Geometry check sheet. Reference: the model listing, model coordinates, mm. A direction names the side the tool comes from. Round coordinates to 2 decimals unless told otherwise and drop trailing zeros. Loops run counter-clockwise (first coordinate to the right, second up) from the corner with the lowest first, then second, coordinate; pieces in that order, holes last. Notation, with made-up numbers: (57.25, -37) -> (80.25, -37) arc R19 cw to (80.25, -26) -> close; hole circle Ø1 at (4.25, 63). An arc over 180 degrees is marked (long way). Use a Markdown table: item, result. Add a question column.
Q1. Gauge pin test, flat ends, axial feed: P1, Ø0.6, axis at x = -0.5, z = 19, coming from the -Y side; P2, Ø0.8, axis at x = 1, z = 17, coming from the -Y side; P3, Ø0.8, axis at x = 4, y = -41, coming from the +Z side. Record the tip position at first contact, or that the pin passes through.
Q2. Set-up check for faces 4 (the face through (0, -42.5, 8)), 5 (the face through (0, -41, 16)), 6 (the face through (25.2, -1.1, 18)), 7 (the face through (25, -2, 9)): record each of +Z, -Z, +X, -X, +Y, -Y from which the full face is reachable in a straight line by a thin tool's end or side.
Q3. Sectioned sample at B-B, the plane x = 21.5. Enter the section's corners in (y, z), then the cut area to 3 significant figures.
Q4. Sectioned sample at C-C, the plane y = 5. Enter the section's corners in (x, z).
Q5. Release check for a two-part mould opening along X. For faces 1 (the face through (-27.5, -1, 10)), 2 (the face through (-25, -2, 9)), 3 (the face through (-27, 13, 20)) record: released by +X, released by -X, zero draft, split by the parting line, or undercut.
Q6. Material ranges on L1, parallel to Y at x = 10, z = 13.75; L2, parallel to X at y = 36, z = 9.75; L3, parallel to Z at x = 25.5, y = -35, recorded low to high.
Q7. Sectioned sample at A-A, the plane z = 11.75. Enter the section's corners in (x, y), then the cut area to 3 significant figures.
```python
from build123d import *

# Parameters (mm, degrees)
F0_W     = 55
F0_H     = 85
F0_W_2   = 50
F0_H_2   = 80
F1_DEPTH = 2
F2_DEPTH = 20
F3_W     = 50
F3_H     = 4
F4_DEPTH = 82.5
F5_W     = 50
F5_H     = 1.5
F5_W_2   = 1
F6_DEPTH = 83.2


with BuildPart() as f1:
    # F0 (on Top) → F1 (new body)
    with BuildSketch(Plane.XY):
        Rectangle(F0_W, F0_H)
        Rectangle(F0_W_2, F0_H_2, mode=Mode.SUBTRACT)
        Rectangle(F0_W_2, F0_H_2)
    extrude(amount=F1_DEPTH)

    # F0 (on Top) → F2 (join)
    with BuildSketch(Plane.XY):
        Rectangle(F0_W, F0_H)
        Rectangle(F0_W_2, F0_H_2, mode=Mode.SUBTRACT)
    extrude(amount=F2_DEPTH)

    # F3 (on face) → F4 (cut, through all)
    with BuildSketch(Plane.XZ.offset(42.5)):
        with Locations((0, 18)):
            Rectangle(F3_W, F3_H)
    extrude(amount=-F4_DEPTH, mode=Mode.SUBTRACT)

    # F5 (on face) → F6 (cut)
    with BuildSketch(Plane.XZ.offset(42.5)):
        with Locations((0, 17.25)):
            Rectangle(F5_W, F5_H)
        with Locations((-25.5, 17.25)):
            Rectangle(F5_W_2, F5_H)
        with Locations((25.5, 17.25)):
            Rectangle(F5_W_2, F5_H)
    extrude(amount=-F6_DEPTH, mode=Mode.SUBTRACT)


solid = f1.part
```
Values:
| question | item | result |
|---|---|---|
| 1 | P1 | y = 40 |
| 1 | P2 | y = 40.7 |
| 1 | P3 | z = 16 |
| 2 | face 4 | +Z, -Z, +X, -X, -Y |
| 2 | face 5 | +Z, -Y |
| 2 | face 6 | -Y |
| 2 | face 7 | +Z |
| 3 | outline | (-42.5, 0) -> (42.5, 0) -> (42.5, 20) -> (40, 20) -> (40, 18) -> (40.7, 18) -> (40.7, 16.5) -> (40, 16.5) -> (40, 2) -> (-40, 2) -> (-40, 16) -> (-42.5, 16) -> close |
| 3 | area | 249 mm^2 |
| 4 | outline | (-27.5, 0) -> (27.5, 0) -> (27.5, 20) -> (25, 20) -> (25, 18) -> (26, 18) -> (26, 16.5) -> (25, 16.5) -> (25, 2) -> (-25, 2) -> (-25, 16.5) -> (-26, 16.5) -> (-26, 18) -> (-25, 18) -> (-25, 20) -> (-27.5, 20) -> close |
| 5 | face 1 | released by -X |
| 5 | face 2 | undercut |
| 5 | face 3 | zero draft |
| 6 | L1 | -42.5 to -40, 40 to 42.5 |
| 6 | L2 | -27.5 to -25, 25 to 27.5 |
| 6 | L3 | 0 to 16.5, 18 to 20 |
| 7 | outline | (-27.5, -42.5) -> (27.5, -42.5) -> (27.5, 42.5) -> (-27.5, 42.5) -> close; hole (-25, -40) -> (25, -40) -> (25, 40) -> (-25, 40) -> close |
| 7 | area | 675 mm^2 |
